Part model, mm, in its own coordinate system. A direction names the side the tool comes from. Coordinates: 2 decimals unless noted, no trailing zeros. Write each loop counter-clockwise with the first axis right and the second up, starting at its lowest first coordinate (ties: lowest second). Pieces come first, ordered by that corner, then holes. Notation, with made-up numbers: (7, 35.25) -> (58, 35.25) arc R15 cw to (58, 60.25) -> close; hole circle Ø3 at (-36.5, -39.75). An arc over 180 degrees is marked (long way). Write item = value, one per line.
from build123d import *

# Parameters (mm, degrees)
SKETCH1_R           = 3.2
SKETCH1_R_2         = 19.5
BOSS_EXTRUDE1_DEPTH = 1.8796
CUT_EXTRUDE1_DEPTH  = 2.8796
SKETCH3_R           = 3.2
BOSS_EXTRUDE2_DEPTH = 1.8796
FILLET1_R           = 6.5
SKETCH4_R           = 1.5
CUT_EXTRUDE2_DEPTH  = 2.8796
FILLET2_R           = 8
SKETCH6_R           = 1.45
CUT_EXTRUDE4_DEPTH  = 2.8796
FILLET3_R           = 3


with BuildPart() as part:
    # Sketch1 → Boss-Extrude1 (new body)
    with BuildSketch(Plane.XY):
        Polygon((0, 36.5), (-10, 35.30709832), (-16, 29), (-56.5, 27.5), (-76.5, 14), (-76.5, -14), (-56.5, -27.5), (-16, -29), (-10, -35.30709832), (0, -36.5), (10, -35.30709832), (16, -29), (56.5, -27.5), (76.5, -14), (76.5, 14), (56.5, 27.5), (16, 29), (10, 35.30709832), align=None)
        with Locations((0, 30)):
            Circle(SKETCH1_R, mode=Mode.SUBTRACT)
        with Locations((-50, 0)):
            Circle(SKETCH1_R_2, mode=Mode.SUBTRACT)
        with Locations((50, 0)):
            Circle(SKETCH1_R_2, mode=Mode.SUBTRACT)
        with Locations((0, -30)):
            Circle(SKETCH1_R, mode=Mode.SUBTRACT)
    extrude(amount=BOSS_EXTRUDE1_DEPTH)

    # Sketch2 → Cut-Extrude1 (cut, through all)
    with BuildSketch(Plane.XY.offset(1.8796)):
        with BuildLine():
            Line((-20.066740906, 20), (20.066740906, 20))
            ThreePointArc((20.066740906, 20), (14, 0), (20.066740906, -20))
            Line((20.066740906, -20), (-20.066740906, -20))
            ThreePointArc((-20.066740906, -20), (-14, 0), (-20.066740906, 20))
        make_face()
    extrude(amount=-CUT_EXTRUDE1_DEPTH, mode=Mode.SUBTRACT)

    # Sketch3 → Boss-Extrude2 (add)
    with BuildSketch(Plane.XY.offset(1.8796)):
        Polygon((-56.5, 27.5), (-65, 32.5), (-80.3, 31), (-73.537037037, 16), align=None)
        with Locations((-70.5, 25.5)):
            Circle(SKETCH3_R, mode=Mode.SUBTRACT)
        Polygon((73.537037037, 16), (56.5, 27.5), (65, 32.5), (80.3, 31), align=None)
        with Locations((70.5, 25.5)):
            Circle(SKETCH3_R, mode=Mode.SUBTRACT)
        Polygon((56.5, -27.5), (65, -32.5), (80.3, -31), (73.537037037, -16), align=None)
        with Locations((70.5, -25.5)):
            Circle(SKETCH3_R, mode=Mode.SUBTRACT)
        Polygon((-73.537037037, -16), (-56.5, -27.5), (-65, -32.5), (-80.3, -31), align=None)
        with Locations((-70.5, -25.5)):
            Circle(SKETCH3_R, mode=Mode.SUBTRACT)
    extrude(amount=-BOSS_EXTRUDE2_DEPTH)

    # Fillet1
    fillet1_edges = [part.edges().sort_by_distance(p)[0] for p in [
        (80.3, -31, 0.9398),
        (-80.3, -31, 0.9398),
        (-80.3, 31, 0.9398),
        (80.3, 31, 0.9398),
    ]]
    fillet(fillet1_edges, radius=FILLET1_R)

    # Sketch4 → Cut-Extrude2 (cut, through all)
    with BuildSketch(Plane.XY.offset(1.8796)):
        with Locations((-50, 23.75)):
            Circle(SKETCH4_R)
        with Locations((-70.56810334, 11.875)):
            Circle(SKETCH4_R)
        with Locations((-70.56810334, -11.875)):
            Circle(SKETCH4_R)
        with Locations((-50, -23.75)):
            Circle(SKETCH4_R)
        with Locations((-29.43189666, -11.875)):
            Circle(SKETCH4_R)
        with Locations((-29.43189666, 11.875)):
            Circle(SKETCH4_R)
        with Locations((29.43189666, 11.875)):
            Circle(SKETCH4_R)
        with Locations((29.43189666, -11.875)):
            Circle(SKETCH4_R)
        with Locations((50, -23.75)):
            Circle(SKETCH4_R)
        with Locations((70.56810334, -11.875)):
            Circle(SKETCH4_R)
        with Locations((70.56810334, 11.875)):
            Circle(SKETCH4_R)
        with Locations((50, 23.75)):
            Circle(SKETCH4_R)
    extrude(amount=-CUT_EXTRUDE2_DEPTH, mode=Mode.SUBTRACT)

    # Fillet2
    fillet2_edges = [part.edges().sort_by_distance(p)[0] for p in [
        (-20.066740906, -20, 0.9398),
        (-20.066740906, 20, 0.9398),
        (20.066740906, 20, 0.9398),
        (20.066740906, -20, 0.9398),
    ]]
    fillet(fillet2_edges, radius=FILLET2_R)

    # Sketch6 → Cut-Extrude4 (cut, through all)
    with BuildSketch(Plane(origin=(0, 0, 0), x_dir=(-1, 0, 0), z_dir=(0, 0, -1))):
        with Locations((8.25, 24.5)):
            Circle(SKETCH6_R)
        with Locations((-8.25, 24.5)):
            Circle(SKETCH6_R)
        with Locations((-8.25, -24.5)):
            Circle(SKETCH6_R)
        with Locations((8.25, -24.5)):
            Circle(SKETCH6_R)
    extrude(amount=-CUT_EXTRUDE4_DEPTH, mode=Mode.SUBTRACT)

    # Fillet3
    fillet3_edges = [part.edges().sort_by_distance(p)[0] for p in [
        (65, -32.5, 0.9398),
        (-65, -32.5, 0.9398),
        (10, 35.30709832, 0.9398),
        (16, 29, 0.9398),
        (56.5, 27.5, 0.9398),
        (56.5, -27.5, 0.9398),
        (16, -29, 0.9398),
        (10, -35.30709832, 0.9398),
        (0, -36.5, 0.9398),
        (-10, -35.30709832, 0.9398),
        (-16, -29, 0.9398),
        (-56.5, -27.5, 0.9398),
        (-56.5, 27.5, 0.9398),
        (-16, 29, 0.9398),
        (-10, 35.30709832, 0.9398),
        (0, 36.5, 0.9398),
        (-65, 32.5, 0.9398),
        (65, 32.5, 0.9398),
    ]]
    fillet(fillet3_edges, radius=FILLET3_R)


solid = part.part
Q1. Probe line 1 (Y direction, x = 50, z = 1.45); line 2 (X direction, y = 8, z = 0.9); line 3 (X direction, y = 6.5, z = 1.8). List the from-to ranges inside material, lowest first. Write a range as from..to.
Model answer:
line_1 = -27.74..-25.25, -22.25..-19.5, 19.5..22.25, 25.25..27.74
line_2 = -76.5..-67.78, -32.22..-14.9, 14.9..32.22, 67.78..76.5
line_3 = -76.5..-68.38, -31.62..-14.59, 14.59..31.62, 68.38..76.5
Q2. Saw through at C-C on x = -23.5. Give the cut face in (y, z), and give its area (3 significant figures).
Model answer:
outline = (-28.72, 0) -> (28.72, 0) -> (28.72, 1.88) -> (-28.72, 1.88) -> close
area = 108 mm²
Q3. Which spindle directions (+Z, -Z, +X, -X, +Y, -Y) get a long thin tool onto all of the face, cutting with end or side? Do faces 5 (the face through (-7.1, 23.62, 0.93)), 6 (the face through (-60.659, -29.946, 0.953)), 7 (the face through (75.08, -19.42, 0.95)). Say none if no direction does.
Model answer:
face_5 = +Z, -Z
face_6 = +Z, -Z, -Y
face_7 = +Z, -Z, +X
Q4. Mould opens along Y. For faces 1 (the face through (-75.08, -19.42, 0.95)), 2 (the face through (12.982, 32.172, 0.927)), 3 (the face through (-69.14, 12.33, 0.95)), 4 (the face through (-12.982, -32.172, 0.927)) say: released by +Y, released by -Y, zero draft, split by the parting line, or undercut.
Model answer:
face_1 = undercut
face_2 = released by +Y
face_3 = undercut
face_4 = released by -Y
Q5. Saw through at A-A on y = 0. Give the cut face in (x, z), and give its area (3 significant figures).
Model answer:
outline = (-76.5, 0) -> (-69.5, 0) -> (-69.5, 1.88) -> (-76.5, 1.88) -> close; (-30.5, 0) -> (-14, 0) -> (-14, 1.88) -> (-30.5, 1.88) -> close; (14, 0) -> (30.5, 0) -> (30.5, 1.88) -> (14, 1.88) -> close; (69.5, 0) -> (76.5, 0) -> (76.5, 1.88) -> (69.5, 1.88) -> close
area = 88.3 mm²
Q6. Saw through at B-B on x = -46.5. Give the cut face in (y, z).
Model answer:
outline = (-27.87, 0) -> (-19.18, 0) -> (-19.18, 1.88) -> (-27.87, 1.88) -> close; (19.18, 0) -> (27.87, 0) -> (27.87, 1.88) -> (19.18, 1.88) -> close
Q7. Pin check, flat tips, straight feed: pin 1 (8.5 mm diameter, centred on x = 70.5, y = -25.5, fed in from -Z); pin 2 (1 mm diameter, centred on x = 15.5, z = 0, fed in from -Y). Stop position of each tip, or through.
Model answer:
pin_1 = 0
pin_2 = -30.05
